from build123d import *

# Parameters (mm, degrees)
SKETCH_W        = 12.7
SKETCH_H        = 45.5
PAD_DEPTH       = 600
SKETCH001_R     = 3
HOLE_DEPTH      = 25
CHAMFER_SIZE    = 1
CHAMFER001_SIZE = 1


with BuildPart() as part:
    # Sketch → Pad (new body)
    with BuildSketch(Plane.XZ):
        with Locations((6.35, 22.75)):
            Rectangle(SKETCH_W, SKETCH_H)
    extrude(amount=-PAD_DEPTH)

    # Sketch001 (on Face4 of Pad) → Hole (cut)
    with BuildSketch(Plane(origin=(0, 0, 0), x_dir=(0, 0, -1), z_dir=(-1, 0, 0))):
        with Locations((-22.75, -51)):
            Circle(SKETCH001_R)
        with Locations((-22.75, -33.5)):
            Circle(SKETCH001_R)
        with Locations((-22.75, -513.5)):
            Circle(SKETCH001_R)
    extrude(amount=-HOLE_DEPTH, mode=Mode.SUBTRACT)

    # Chamfer
    chamfer_edges = [part.edges().sort_by_distance(p)[0] for p in [
        (0, 516.5, 22.75),
    ]]
    chamfer(chamfer_edges, length=CHAMFER_SIZE)

    # Chamfer001
    chamfer001_edges = [part.edges().sort_by_distance(p)[0] for p in [
        (12.7, 36.5, 22.75),
        (12.7, 516.5, 22.75),
    ]]
    chamfer(chamfer001_edges, length=CHAMFER001_SIZE)


solid = part.part
Here's how the part is built. I have some questions about the finished solid (model axes, mm). Give positions to 0.01 mm unless a question says otherwise; leave off trailing zeros. One line per item, written item: value. Start each with the question number.
1. Will these pins go through, and if not, where does the flat tip stop? pin 1 Ø5 at (y, z) = (33.5, 22.75) entering from +X; pin 2 Ø5 at (x, y) = (10.5, 381) entering from -Z.
2. We'd pull the mould along Z, two halves only. Please class faces 1 (the face through (12.7, 296, 22)), 2 (the face through (6, 296, 45.5)), 3 (the face through (6, 296, 0)): released by +Z, released by -Z, zero draft, split by the parting line, or undercut.
3. I need wall thicknesses on probe 1 along Y at (x, z) = (9, 22.75); probe 2 along Z at (x, y) = (3.75, 33.5); probe 3 along Y at (x, z) = (3.25, 24.5). Which ranges of each line are inside material? Lowest first, please. Write a range as from..to.
Values follow:
1. pin 1: passes through
1. pin 2: stops at z = 0
2. face 1: zero draft
2. face 2: released by +Z
2. face 3: released by -Z
3. probe 1: y = 0..30.5, 36.5..48, 54..510.5, 516.5..600
3. probe 2: z = 0..19.75, 25.75..45.5
3. probe 3: y = 0..31.06, 35.94..48.56, 53.44..511.06, 515.94..600
